from build123d import *

# Parameters (mm, degrees)
CUT_EXTRUDE1_DEPTH = 3.81
SKETCH6_R          = 1.5
CUT_EXTRUDE2_DEPTH = 14.508000035


with BuildPart() as part:
    # Sketch2 → Main Revolve (revolve)
    with BuildSketch(Plane(origin=(0, 0, 0), x_dir=(1, 0, 0), z_dir=(0, 1, 0))):
        with BuildLine():
            Line((4, 8.05052812), (4, 9.32052812))
            Line((4, 9.32052812), (0, 9.32052812))
            add(Edge.make_bspline(
                [(-11.730000035, 25.4), (-11.939852155, 16.185984948), (-5.767624941, 10.573485752), (0, 9.32052812)],
                knots=[0, 0, 0, 0, 1, 1, 1, 1], degree=3))
            Line((-11.730000035, 25.4), (13.000000035, 25.4))
            Line((13.000000035, 25.4), (13.000000035, 27.94))
            Line((13.000000035, 27.94), (-13.000000035, 27.94))
            Line((-13.000000035, 27.94), (-13.000000035, 25.4))
            add(Edge.make_bspline(
                [(-0.508, 8.128), (-13.159061445, 7.336688862), (-13.000000035, 25.4)],
                knots=[0, 0, 0, 1, 1, 1], degree=2))
            Line((-0.508, 8.128), (-0.508, 0))
            Line((-0.508, 0), (4, 0))
            Line((4, 0), (4, 8.05052812))
        make_face()
    revolve(axis=Axis((4, 0, 0), (-1, 0, 0)))

    # Sketch5 → Cut-Extrude1 (cut)
    with BuildSketch(Plane(origin=(4, 0, 0), x_dir=(0, 0, -1), z_dir=(1, 0, 0))):
        Polygon((6.92820323, 0), (3.464101615, 6), (-3.464101615, 6), (-6.92820323, 0), (-3.464101615, -6), (3.464101615, -6), align=None)
    extrude(amount=-CUT_EXTRUDE1_DEPTH, mode=Mode.SUBTRACT)

    # Sketch6 → Cut-Extrude2 (cut, through all)
    with BuildSketch(Plane.ZY.offset(0.508)):
        Circle(SKETCH6_R)
    extrude(amount=-CUT_EXTRUDE2_DEPTH, mode=Mode.SUBTRACT)


solid = part.part
Read the model definition and answer for the solid it produces. Units are mm, in the model's axes. A direction names the side the tool comes from. Round coordinates to 2 decimals unless told otherwise and drop trailing zeros. Write each loop counter-clockwise with the first axis right and the second up, starting at its lowest first coordinate (ties: lowest second). Pieces come first, ordered by that corner, then holes.
Q1. Straight lines are drawn through the part: line 1 (Y direction, x = 0, z = 0); line 2 (Y direction, x = 0.5, z = 0); line 3 (Z direction, x = 2, y = 0). For each, find the intervals that lie inside material, in ascending order.
Values:
line 1: y = -27.94 to -25.4, -9.32 to -1.5, 1.5 to 9.32, 25.4 to 27.94
line 2: y = -27.94 to -25.4, -9.32 to -6, 6 to 9.32, 25.4 to 27.94
line 3: z = -27.94 to -25.4, -9.32 to -6.93, 6.93 to 9.32, 25.4 to 27.94
Q2. Flat-ended cylindrical pins translate along their axes: P1, Ø3.5, axis at y = 3, z = -3, coming from the +X side; P2, Ø4, axis at x = 10, y = -3, coming from the -Z side; P3, Ø1.5, axis at x = 8.5, z = 6.5, coming from the +Y side. Find the tip coordinate at first contact, or state that the pin passes through.
Values:
P1: stops at x = 0.19
P2: stops at z = -27.92
P3: stops at y = 27.34
Q3. The mould has two halves that part along Y. Classify faces 1 (the face through (2, -6, 0)), 2 (the face through (-0.18, -27.7, 3.64)), 3 (the face through (13, 25, 6)), 4 (the face through (2, 6, 0)): released by +Y, released by -Y, zero draft, split by the parting line, or undercut.
Values:
face 1: undercut
face 2: split by the parting line
face 3: zero draft
face 4: undercut
Q4. Find section A-A on x = 10. Determine the outline of the cut face in (y, z).
Values:
outline: circle Ø55.88 at (0, 0); hole circle Ø50.8 at (0, 0)
Q5. A tool of negligible diameter and unlimited length cuts with its end or side. For faces 5 (the face through (0.19, 1.4, -1.4)), 6 (the face through (-13, 25, -6)), from which of +Z, -Z, +X, -X, +Y, -Y can it reach the whole face along a straight path? Write none if from no direction.
Values:
face 5: +X
face 6: +Z, -Z, -X, +Y, -Y
